For this review, take the finished solid that the model builds, in its own axes (mm). Give positions to 0.01 mm unless a question says otherwise; leave off trailing zeros. Order: outer loops, then holes, each group sorted by start corner. A loop starts at its lowest first (then second) coordinate and runs counter-clockwise, first axis right, second up.
from build123d import *

# Parameters (mm, degrees)
SKETCH1_R           = 75
SKETCH1_R_2         = 10
BOSS_EXTRUDE1_DEPTH = 10


with BuildPart() as part:
    # Sketch1 → Boss-Extrude1 (new body)
    with BuildSketch(Plane.XY):
        Circle(SKETCH1_R)
        with Locations((0, 53.737864078)):
            Circle(SKETCH1_R_2, mode=Mode.SUBTRACT)
        with Locations((37.998408096, 37.998408096)):
            Circle(SKETCH1_R_2, mode=Mode.SUBTRACT)
        with Locations((53.737864078, 0)):
            Circle(SKETCH1_R_2, mode=Mode.SUBTRACT)
        with Locations((37.998408096, -37.998408096)):
            Circle(SKETCH1_R_2, mode=Mode.SUBTRACT)
        with Locations((0, -53.737864078)):
            Circle(SKETCH1_R_2, mode=Mode.SUBTRACT)
        with Locations((-37.998408096, -37.998408096)):
            Circle(SKETCH1_R_2, mode=Mode.SUBTRACT)
        with Locations((-53.737864078, 0)):
            Circle(SKETCH1_R_2, mode=Mode.SUBTRACT)
        with Locations((-37.998408096, 37.998408096)):
            Circle(SKETCH1_R_2, mode=Mode.SUBTRACT)
    extrude(amount=BOSS_EXTRUDE1_DEPTH)


solid = part.part
1) We need section D-D on z = 7.5. Count the separate pieces of the cut face and the enclosed holes in it, then the cut area to 3 significant figures.
Answer sheet:
separate pieces: 1
enclosed holes: 8
area: 15,200 mm2
2) Clearance check with flat-ended pins moving along their axes: pin 1 (16 mm diameter, centred on x = -38, y = 38, fed in from -Z); pin 2 (1.5 mm diameter, centred on y = -53.5, z = 2, fed in from +X); pin 3 (8 mm diameter, centred on x = 15.5, y = -0.5, fed in from -Z); pin 4 (1 mm diameter, centred on x = -52, z = 8.5, fed in from -Y). State where each tip first meets the part, or that it passes through.
Answer sheet:
pin 1: passes through
pin 2: stops at x = 53.31
pin 3: stops at z = 0
pin 4: stops at y = -54.52
3) To check wall thickness, follow line 1 (X direction, y = 47, z = 6); line 2 (Y direction, x = 9, z = 0.5); line 3 (X direction, y = 1, z = 4). State the ranges of each line that lie inside material, in increasing order.
Answer sheet:
line 1: x = -58.45 to -42.35, -33.64 to -7.39, 7.39 to 33.64, 42.35 to 58.45
line 2: y = -74.46 to -58.1, -49.38 to 49.38, 58.1 to 74.46
line 3: x = -74.99 to -63.69, -43.79 to 43.79, 63.69 to 74.99
4) Draft analysis for pull direction X (two halves, no side actions). For faces 1 (the face through (-28.76, 34.17, 4.93)), 2 (the face through (-1, 1, 10)), 3 (the face through (63.276, 3.004, 4.93)), 4 (the face through (-9.764, 74.362, 4.93)), state which applies: +X half, -X half, draft (parallel to the pull), parting line (faces both ways), or undercut.
Answer sheet:
face 1: undercut
face 2: draft
face 3: undercut
face 4: parting line
5) We need section A-A on y = 0. Give the boundary of the cut face in (x, z).
Answer sheet:
outline: (-75, 0) - (-63.74, 0) - (-63.74, 10) - (-75, 10) - close; (-43.74, 0) - (43.74, 0) - (43.74, 10) - (-43.74, 10) - close; (63.74, 0) - (75, 0) - (75, 10) - (63.74, 10) - close
6) We need section C-C on y = -56. Give the boundary of the cut face in (x, z), then the cut area to 3 significant figures.
Answer sheet:
outline: (-49.89, 0) - (-9.74, 0) - (-9.74, 10) - (-49.89, 10) - close; (9.74, 0) - (49.89, 0) - (49.89, 10) - (9.74, 10) - close
area: 803 mm2
